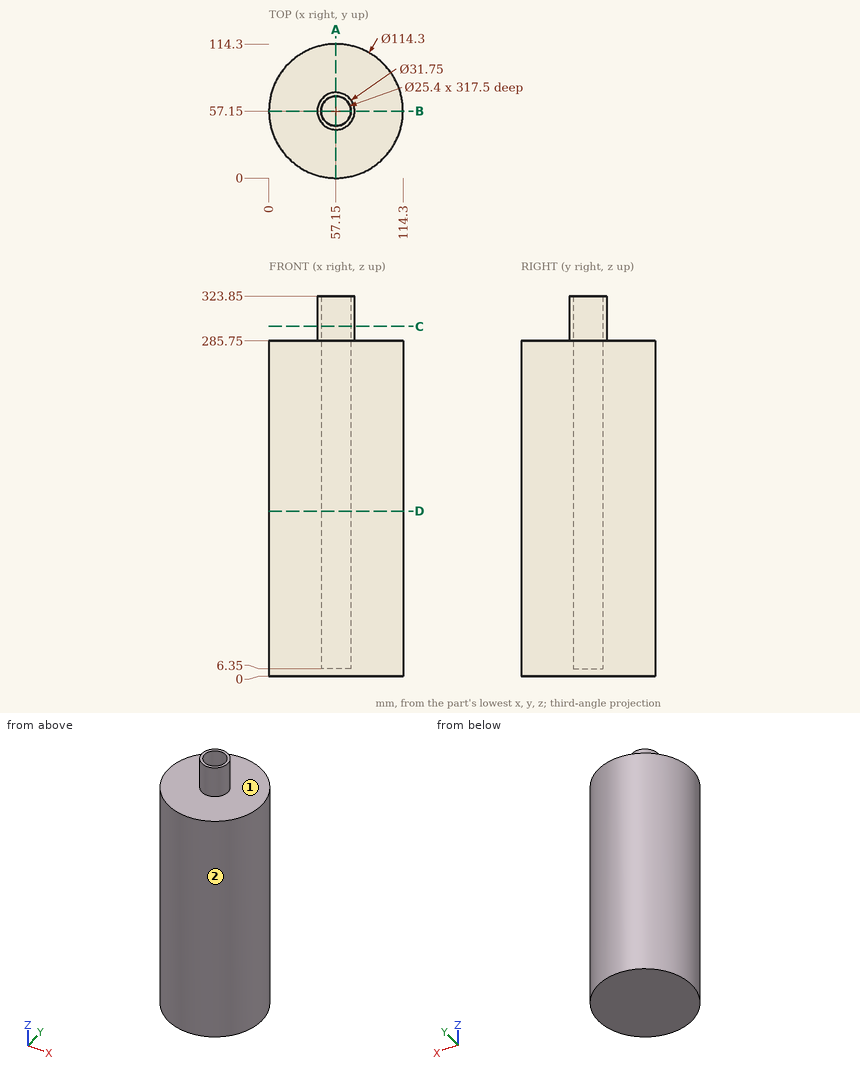
Can you work these out from the drawing? Everything is in mm from the part's minimum corner. A direction names the side the tool comes from. Round coordinates to 2 decimals unless told otherwise and drop trailing zeros. Loops run counter-clockwise (first coordinate to the right, second up) from the corner with the lowest first, then second, coordinate; pieces in that order, holes last. Notation, with made-up numbers: (20, 76) -> (72, 76) arc R19 ccw to (72, 98) -> close; hole circle Ø3 at (-14.5, 23.25). An arc over 180 degrees is marked (long way). Put each result on its own line as item: value.
Q1. I want a section at A-A on x = 57.15. Write out the boundary of the cut face in (y, z) (3 decimals), and give its area (3 significant figures).
Checks:
outline: (0, 0) -> (114.3, 0) -> (114.3, 285.75) -> (73.025, 285.75) -> (73.025, 323.85) -> (69.85, 323.85) -> (69.85, 6.35) -> (44.45, 6.35) -> (44.45, 323.85) -> (41.275, 323.85) -> (41.275, 285.75) -> (0, 285.75) -> close
area: 25,800 mm2
Q2. For pin 1 Ø5 at (y, z) = (12.5, 195) entering from -X; pin 2 Ø1 at (y, z) = (18.5, 234) entering from +X; pin 3 Ø20.5 at (x, y) = (57.15, 57.15) entering from +Z; pin 4 Ø5 at (x, y) = (81, 29.5) entering from -Z, each with a flat end and sliding along its axis, tell me the tip position at first contact or that it passes through.
Checks:
pin 1: x = 18.56
pin 2: x = 99.7
pin 3: z = 6.35
pin 4: z = 0
Q3. Please list where these lines run through material, in increasing order: line 1 (Y direction, x = 57.15, z = 216.5); line 2 (Z direction, x = 54, y = 45). Write a range as from..to.
Checks:
line 1: 0..44.45, 69.85..114.3
line 2: 0..6.35
Q4. Which directions (+Z, -Z, +X, -X, +Y, -Y) give clear straight access to the entire face, cutting with the end or side of a thin tool? Please do the marked faces 1 and 2.
Checks:
face 1: +Z
face 2: +Z, -Z
Q5. I want a section at D-D on z = 140.5. Write out the boundary of the cut face in (x, y).
Checks:
outline: circle Ø114.3 at (57.15, 57.15); hole circle Ø25.4 at (57.15, 57.15)
Q6. I want a section at C-C on z = 298. Write out the boundary of the cut face in (x, y) (3 decimals).
Checks:
outline: circle Ø31.75 at (57.15, 57.15); hole circle Ø25.4 at (57.15, 57.15)
